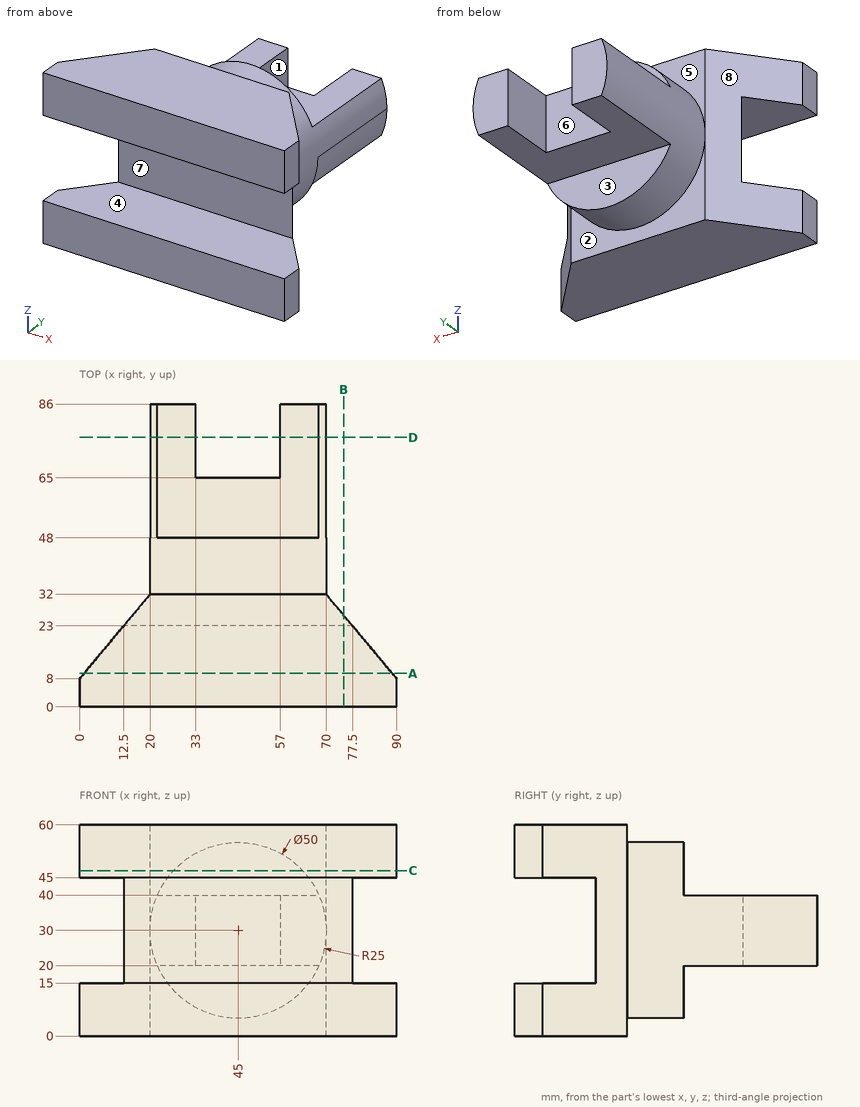
Answer from the drawing. Dimensions are ordinates in mm from the lowest x, y and z of the part. A direction names the side the tool comes from. Give positions to 0.01 mm unless a question says otherwise; leave off trailing zeros. Order: outer loops, then holes, each group sorted by start corner. A loop starts at its lowest first (then second) coordinate and runs counter-clockwise, first axis right, second up. Notation, with made-up numbers: (29, -2.5) -> (42, -2.5) arc R19 cw to (42, 2.5) -> close; hole circle Ø6 at (31.5, 8.25). An arc over 180 degrees is marked (long way). One line per item, written item: value. Start each with the question number.
(1) Straight lines are drawn through the part: L1, parallel to Z at x = 41.5, y = 6; L2, parallel to Z at x = 44, y = 60.5; L3, parallel to Y at x = 42, z = 18.5. For each, find the intervals that lie inside material, in ascending order.
(2) The part is cut by section D-D (y = 76.5). Determine the outline of the cut face in (x, z), and give its area (3 significant figures).
(3) The part is cut by section C-C (z = 47). Determine the outline of the cut face in (x, y).
(4) Flat-ended cylindrical pins translate along their axes: P1, Ø12, axis at x = 53, y = 39, coming from the +Z side; P2, Ø16.5, axis at x = 44.5, z = 48.5, coming from the +Y side; P3, Ø5, axis at x = 14, z = 41, coming from the +Y side; P4, Ø12, axis at y = 74, z = 51.5, coming from the +X side. Find the tip coordinate at first contact, or state that the pin passes through.
(5) A tool of negligible diameter and unlimited length cuts with its end or side. For the marked faces 1, 2, 3, 4 and 5, from which of +Z, -Z, +X, -X, +Y, -Y can it reach the whole face along a straight path? Write none if from no direction.
(6) For a pull along X with two mould halves and no side action, classify the marked faces 6, 7 and 8 as released by +X, released by -X, zero draft, split by the parting line, or undercut.
(7) The part is cut by section B-B (x = 75). Determine the outline of the cut face in (y, z).
(8) The part is cut by section A-A (y = 9.5). Determine the outline of the cut face in (x, z).
Taken from the geometry:
1. L1: 0 to 15, 45 to 60
1. L2: 20 to 40
1. L3: 23 to 48
2. outline: (22.09, 20) -> (33, 20) -> (33, 40) -> (22.09, 40) arc R25 ccw to start; (57, 20) -> (67.91, 20) arc R25 ccw to (67.91, 40) -> (57, 40) -> close
2. area: 493 mm^2
3. outline: (0, 0) -> (90, 0) -> (90, 8) -> (70, 32) -> (63.33, 32) -> (63.33, 48) -> (26.67, 48) -> (26.67, 32) -> (20, 32) -> (0, 8) -> close
4. P1: z = 54.92
4. P2: y = 48
4. P3: y = 27.8
4. P4: through
5. face 1: +Z, -Z, +Y
5. face 2: -Z, +Y
5. face 3: -Z, +X, -X, +Y
5. face 4: +X, -X, -Y
5. face 5: +Z, +Y
6. face 6: undercut
6. face 7: zero draft
6. face 8: released by -X
7. outline: (0, 0) -> (26, 0) -> (26, 60) -> (0, 60) -> (0, 45) -> (23, 45) -> (23, 15) -> (0, 15) -> close
8. outline: (1.25, 0) -> (88.75, 0) -> (88.75, 15) -> (1.25, 15) -> close; (1.25, 45) -> (88.75, 45) -> (88.75, 60) -> (1.25, 60) -> close
